Check sheet for the modelled part. Datum: model origin and axes. Units: mm. A direction names the side the tool comes from. Round coordinates to 2 decimals unless told otherwise and drop trailing zeros. Order: outer loops, then holes, each group sorted by start corner. A loop starts at its lowest first (then second) coordinate and runs counter-clockwise, first axis right, second up. Notation, with made-up numbers: (-20, 32.25) -> (-3, 32.25) arc R28 cw to (-3, 66.25) -> close; hole circle Ø3 at (19.25, 53.5). An arc over 180 degrees is marked (long way). Use CSV: the item, a comma, the result in double quotes.
```python
from build123d import *

# Parameters (mm, degrees)
SKETCH1_W           = 60
SKETCH1_H           = 56.5
SKETCH1_H_2         = 30
BOSS_EXTRUDE1_DEPTH = 10
SKETCH3_W           = 60
SKETCH3_H           = 10
BOSS_EXTRUDE2_DEPTH = 40
SKETCH4_W           = 9
SKETCH4_H           = 5
BOSS_EXTRUDE3_DEPTH = 40
CUT_EXTRUDE1_REACH  = 88.5
SKETCH5_R           = 1.5


with BuildPart() as part:
    # Sketch1 → Boss-Extrude1 (new body)
    with BuildSketch(Plane(origin=(0, 0, 0), x_dir=(0, 0, -1), z_dir=(1, 0, 0))):
        with Locations((0, 28.25)):
            Rectangle(SKETCH1_W, SKETCH1_H)
        with Locations((0, -15)):
            Rectangle(SKETCH1_W, SKETCH1_H_2)
        with BuildLine():
            ThreePointArc((-20, -21.7), (-23.2, -18.5), (-20, -15.3))
            Line((-20, -15.3), (20, -15.3))
            ThreePointArc((20, -15.3), (22.2627417, -16.2372583), (23.2, -18.5))
            ThreePointArc((23.2, -18.5), (22.2627417, -20.7627417), (20, -21.7))
            Line((20, -21.7), (-20, -21.7))
        make_face(mode=Mode.SUBTRACT)
        with BuildLine():
            ThreePointArc((-20, -11.7), (-23.2, -8.5), (-20, -5.3))
            Line((-20, -5.3), (20, -5.3))
            ThreePointArc((20, -5.3), (22.2627417, -6.2372583), (23.2, -8.5))
            ThreePointArc((23.2, -8.5), (22.2627417, -10.7627417), (20, -11.7))
            Line((20, -11.7), (-20, -11.7))
        make_face(mode=Mode.SUBTRACT)
    extrude(amount=BOSS_EXTRUDE1_DEPTH)

    # Sketch3 → Boss-Extrude2 (add)
    with BuildSketch(Plane.ZY):
        with Locations((0, 5)):
            Rectangle(SKETCH3_W, SKETCH3_H)
    extrude(amount=BOSS_EXTRUDE2_DEPTH)

    # Sketch4 → Boss-Extrude3 (add)
    with BuildSketch(Plane.ZY):
        with Locations((-15.5, 54)):
            Rectangle(SKETCH4_W, SKETCH4_H)
        with Locations((15.5, 54)):
            Rectangle(SKETCH4_W, SKETCH4_H)
    extrude(amount=BOSS_EXTRUDE3_DEPTH)

    # Sketch5 → Cut-Extrude1 (cut, up to next)
    with BuildSketch(Plane(origin=(0, 56.5, 0), x_dir=(1, 0, 0), z_dir=(0, 1, 0)), mode=Mode.PRIVATE) as cut_extrude1_sk1:
        with Locations((-5.5, 15.5)):
            Circle(SKETCH5_R)
    cut_extrude1_tool1 = extrude(cut_extrude1_sk1.sketch, amount=-CUT_EXTRUDE1_REACH, mode=Mode.PRIVATE) & part.part
    add(cut_extrude1_tool1.solids().sort_by_distance((-5.5, 56.5, -15.5))[0], mode=Mode.SUBTRACT)
    # Sketch5 → Cut-Extrude1 (cut, up to next)
    with BuildSketch(Plane(origin=(0, 56.5, 0), x_dir=(1, 0, 0), z_dir=(0, 1, 0)), mode=Mode.PRIVATE) as cut_extrude1_sk2:
        with Locations((-36.5, 15.5)):
            Circle(SKETCH5_R)
    cut_extrude1_tool2 = extrude(cut_extrude1_sk2.sketch, amount=-CUT_EXTRUDE1_REACH, mode=Mode.PRIVATE) & part.part
    add(cut_extrude1_tool2.solids().sort_by_distance((-36.5, 56.5, -15.5))[0], mode=Mode.SUBTRACT)
    # Sketch5 → Cut-Extrude1 (cut, up to next)
    with BuildSketch(Plane(origin=(0, 56.5, 0), x_dir=(1, 0, 0), z_dir=(0, 1, 0)), mode=Mode.PRIVATE) as cut_extrude1_sk3:
        with Locations((-5.5, -15.5)):
            Circle(SKETCH5_R)
    cut_extrude1_tool3 = extrude(cut_extrude1_sk3.sketch, amount=-CUT_EXTRUDE1_REACH, mode=Mode.PRIVATE) & part.part
    add(cut_extrude1_tool3.solids().sort_by_distance((-5.5, 56.5, 15.5))[0], mode=Mode.SUBTRACT)
    # Sketch5 → Cut-Extrude1 (cut, up to next)
    with BuildSketch(Plane(origin=(0, 56.5, 0), x_dir=(1, 0, 0), z_dir=(0, 1, 0)), mode=Mode.PRIVATE) as cut_extrude1_sk4:
        with Locations((-36.5, -15.5)):
            Circle(SKETCH5_R)
    cut_extrude1_tool4 = extrude(cut_extrude1_sk4.sketch, amount=-CUT_EXTRUDE1_REACH, mode=Mode.PRIVATE) & part.part
    add(cut_extrude1_tool4.solids().sort_by_distance((-36.5, 56.5, 15.5))[0], mode=Mode.SUBTRACT)


solid = part.part
```
Q1. Access from +Z, -Z, +X, -X, +Y, -Y to the whole of each face (thin tool, end or side, straight path). Record for faces 5 (the face through (-37.7, 54, -14.6)), 6 (the face through (-20, 0, 0)), 7 (the face through (-20, 54, 11)), 8 (the face through (4.9, -18.6, 23.2)).
Result sheet:
face 5,"+Y"
face 6,"+Z, -Z, -X, -Y"
face 7,"-X, +Y"
face 8,"+X, -X"
Q2. Sectioned sample at B-B, the plane x = -9. Enter the section's corners in (y, z).
Result sheet:
outline,"(0, -30) -> (10, -30) -> (10, 30) -> (0, 30) -> close; (51.5, -20) -> (56.5, -20) -> (56.5, -11) -> (51.5, -11) -> close; (51.5, 11) -> (56.5, 11) -> (56.5, 20) -> (51.5, 20) -> close"
Q3. Mould release check, pull along Z, two halves, no side actions. Record for faces 1 (the face through (-40, 54, 15)), 2 (the face through (-37.7, 54, 16.4)), 3 (the face through (-20, 54, -20)), 4 (the face through (-20, 54, 20)): pulls with the +Z half, pulls with the -Z half, needs draft (parallel to the pull), parting line crosses it, or undercut.
Result sheet:
face 1,"needs draft"
face 2,"undercut"
face 3,"pulls with the -Z half"
face 4,"pulls with the +Z half"
Q4. Go/stop test with flat-tipped pins: pin 1 (5.5 mm diameter, centred on x = -14.5, y = 54, fed in from +Z); pin 2 (5 mm diameter, centred on x = -36.5, z = -15.5, fed in from -Y); pin 3 (1.5 mm diameter, centred on y = -19.5, z = -1.5, fed in from -X); pin 4 (2.5 mm diameter, centred on x = -10.5, y = 55, fed in from -Z). Record where each tip stops, or that it passes through.
Result sheet:
pin 1,"stops at z = 20"
pin 2,"stops at y = 0"
pin 3,"passes through"
pin 4,"stops at z = -20"
Q5. Scan lines: L1, parallel to Z at x = -5.5, y = 53.2; L2, parallel to X at y = 53.25, z = 15.5; L3, parallel to Y at x = 7.5, z = 2. Record each from-to range of solid material in increasing order.
Result sheet:
L1,"z = -20 to -17, -14 to -11, 11 to 14, 17 to 20"
L2,"x = -40 to -38, -35 to -7, -4 to 10"
L3,"y = -30 to -21.7, -15.3 to -11.7, -5.3 to 56.5"
Q6. Sectioned sample at C-C, the plane x = -36.5. Enter the section's corners in (y, z), then the cut area to 3 significant figures.
Result sheet:
outline,"(0, -30) -> (10, -30) -> (10, 30) -> (0, 30) -> close; (51.5, -20) -> (56.5, -20) -> (56.5, -17) -> (51.5, -17) -> close; (51.5, -14) -> (56.5, -14) -> (56.5, -11) -> (51.5, -11) -> close; (51.5, 11) -> (56.5, 11) -> (56.5, 14) -> (51.5, 14) -> close; (51.5, 17) -> (56.5, 17) -> (56.5, 20) -> (51.5, 20) -> close"
area,"660 mm^2"
Q7. Sectioned sample at D-D, the plane y = -6.5. Enter the section's corners in (x, z), then the cut area to 3 significant figures.
Result sheet:
outline,"(0, -30) -> (10, -30) -> (10, -22.5) -> (0, -22.5) -> close; (0, 22.5) -> (10, 22.5) -> (10, 30) -> (0, 30) -> close"
area,"150 mm^2"
Q8. Sectioned sample at A-A, the plane z = -15.5. Enter the section's corners in (x, y).
Result sheet:
outline,"(-40, 0) -> (0, 0) -> (0, -5.3) -> (10, -5.3) -> (10, 56.5) -> (-4, 56.5) -> (-4, 51.5) -> (0, 51.5) -> (0, 10) -> (-40, 10) -> close; (-40, 51.5) -> (-38, 51.5) -> (-38, 56.5) -> (-40, 56.5) -> close; (-35, 51.5) -> (-7, 51.5) -> (-7, 56.5) -> (-35, 56.5) -> close; (0, -30) -> (10, -30) -> (10, -21.7) -> (0, -21.7) -> close; (0, -15.3) -> (10, -15.3) -> (10, -11.7) -> (0, -11.7) -> close"
